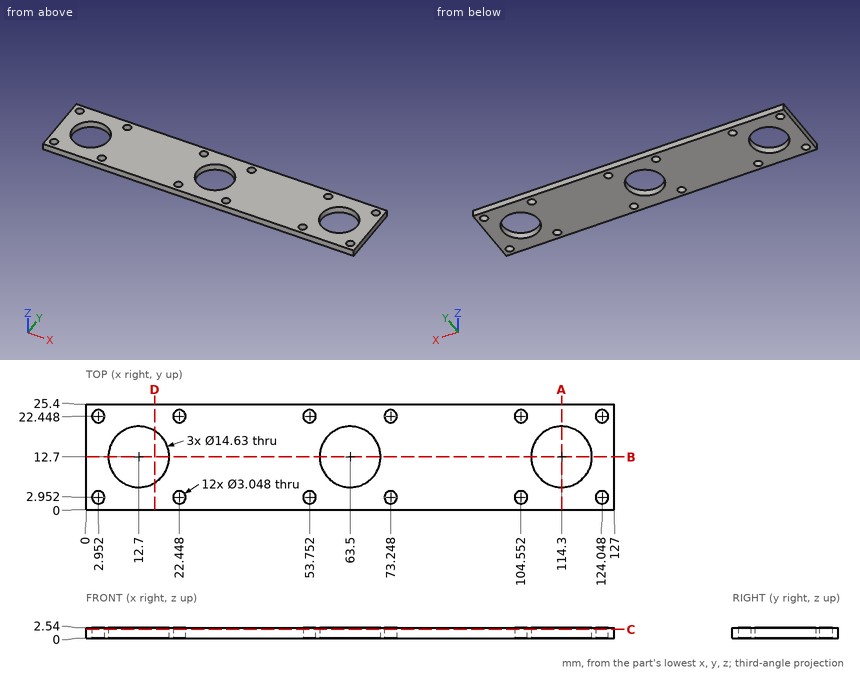
Design review of the part shown in the three views and the two pictorial views. Dimensions are in mm from the part's minimum x, y and z. Coordinates: 2 decimals unless noted, no trailing zeros. Write each loop counter-clockwise with the first axis right and the second up, starting at its lowest first coordinate (ties: lowest second). Pieces come first, ordered by that corner, then holes. Notation, with made-up numbers: (-6.5, 38) -> (6.5, 38) arc R17 cw to (6.5, 63) -> close; hole circle Ø5 at (-4.5, 31.5). An arc over 180 degrees is marked (long way). Answer in a Markdown table with one row per item.
1. We need section C-C, the plane z = 2.15. Give the number of separate pieces and of enclosed holes in the cut face, and give its area (3 significant figures).
Answers below:
| item | result |
|---|---|
| separate pieces | 1 |
| enclosed holes | 15 |
| area | 2,630 mm^2 |
2. Wall thickness on probe 1 along X at (y, z) = (17.75, 0.7); probe 2 along Y at (x, z) = (12.7, 0.55) (1 decimal); probe 3 along X at (y, z) = (8.25, 0.35) (1 decimal): over which ranges is each line inside the solid? List them lowest first. Write a range as [from, to].
Answers below:
| item | result |
|---|---|
| probe 1 | x = [0, 7.41], [17.99, 58.21], [68.79, 109.01], [119.59, 127] |
| probe 2 | y = [0, 5.4], [20, 25.4] |
| probe 3 | x = [0, 6.9], [18.5, 57.7], [69.3, 108.5], [120.1, 127] |
3. Clearance check with flat-ended pins moving along their axes: pin 1 Ø1.8 at (x, y) = (22.45, 2.95) entering from +Z; pin 2 Ø3.5 at (x, y) = (73.25, 22.45) entering from +Z. State where each tip first meets the part, or that it passes through.
Answers below:
| item | result |
|---|---|
| pin 1 | passes through |
| pin 2 | stops at z = 2.54 |
4. We need section D-D, the plane x = 16.5. State the section outline as (y, z) points.
Answers below:
| item | result |
|---|---|
| outline | (0, 0) -> (6.45, 0) -> (6.45, 2.54) -> (0, 2.54) -> close; (18.95, 0) -> (25.4, 0) -> (25.4, 2.54) -> (18.95, 2.54) -> close |
5. We need section B-B, the plane y = 12.7. State the section outline as (x, z) points (1 decimal).
Answers below:
| item | result |
|---|---|
| outline | (0, 0) -> (5.4, 0) -> (5.4, 2.5) -> (0, 2.5) -> close; (20, 0) -> (56.2, 0) -> (56.2, 2.5) -> (20, 2.5) -> close; (70.8, 0) -> (107, 0) -> (107, 2.5) -> (70.8, 2.5) -> close; (121.6, 0) -> (127, 0) -> (127, 2.5) -> (121.6, 2.5) -> close |
6. We need section A-A, the plane x = 114.3. State the section outline as (y, z) points (1 decimal).
Answers below:
| item | result |
|---|---|
| outline | (0, 0) -> (5.4, 0) -> (5.4, 2.5) -> (0, 2.5) -> close; (20, 0) -> (25.4, 0) -> (25.4, 2.5) -> (20, 2.5) -> close |
